Read the model definition and answer for the solid it produces. Units are mm, in the model's axes. A direction names the side the tool comes from. Round coordinates to 2 decimals unless told otherwise and drop trailing zeros. Loops run counter-clockwise (first coordinate to the right, second up) from the corner with the lowest first, then second, coordinate; pieces in that order, holes last. Notation, with made-up numbers: M 87.25,-1 L 99.25,-1 A15 cw 99.25,8 Z; hole C -29,18 d5. An arc over 180 degrees is marked long. Write each question's results on one line, items separated by ' | '.
from build123d import *

# Parameters (mm, degrees)
ESQUISSE3_W        = 75
ESQUISSE3_H        = 60
BOSS_EXTRU_4_DEPTH = 2
ESQUISSE7_R        = 3
ESQUISSE7_R_2      = 1
BOSS_EXTRU_5_DEPTH = 7


with BuildPart() as part:
    # Esquisse3 → Boss.-Extru.4 (new body)
    with BuildSketch(Plane.XY):
        Rectangle(ESQUISSE3_W, ESQUISSE3_H)
    extrude(amount=BOSS_EXTRU_4_DEPTH)

    # Esquisse7 → Boss.-Extru.5 (add)
    with BuildSketch(Plane.XY.offset(2)):
        with Locations((-17, 13.6)):
            Circle(ESQUISSE7_R)
        with Locations((17, 13.6)):
            Circle(ESQUISSE7_R)
        with Locations((7.649218941, -7.4)):
            Circle(ESQUISSE7_R_2)
    extrude(amount=BOSS_EXTRU_5_DEPTH)


solid = part.part
Item 1: The mould has two halves that part along X. Classify faces 1 (the face through (-17.391, 16.574, 5.451)), 2 (the face through (16.609, 16.574, 5.451)), 3 (the face through (17, 14, 9)), 4 (the face through (37.5, 0, 1)): pulls with the +X half, pulls with the -X half, needs draft (parallel to the pull), parting line crosses it, or undercut.
Outcome:
face 1: undercut | face 2: undercut | face 3: needs draft | face 4: pulls with the +X half
Item 2: The part is cut by section B-B (x = -17). Determine the outline of the cut face in (y, z), plus the area to 3 significant figures.
Outcome:
outline: M -30,0 L 30,0 L 30,2 L 16.6,2 L 16.6,9 L 10.6,9 L 10.6,2 L -30,2 Z | area: 162 mm2
Item 3: For faces 5 (the face through (7.52, -6.41, 5.45)), 6 (the face through (-37.5, 0, 1)), determine the directions among +Z, -Z, +X, -X, +Y, -Y from which every point of the face is accessible in a straight line to the end or side of a thin tool.
Outcome:
face 5: +Z | face 6: +Z, -Z, -X, +Y, -Y
Item 4: Straight lines are drawn through the part: line 1 (Z direction, x = 8, y = -21.5); line 2 (X direction, y = 13, z = 5.5); line 3 (Y direction, x = 19, z = 4.25). For each, find the intervals that lie inside material, in ascending order.
Outcome:
line 1: z = 0 to 2 | line 2: x = -19.94 to -14.06, 14.06 to 19.94 | line 3: y = 11.36 to 15.84
Item 5: A flat-ended cylindrical pin translates along its axis: pin 1 (3 mm diameter, centred on x = 5.5, z = 7, fed in from -Y). Find the tip coordinate at first contact, or state that the pin passes through.
Outcome:
pin 1: stops at y = -8.16
Item 6: The part is cut by section D-D (y = 13.6). Determine the outline of the cut face in (x, z).
Outcome:
outline: M -37.5,0 L 37.5,0 L 37.5,2 L 20,2 L 20,9 L 14,9 L 14,2 L -14,2 L -14,9 L -20,9 L -20,2 L -37.5,2 Z
Item 7: The part is cut by section A-A (y = -7.4). Determine the outline of the cut face in (x, z).
Outcome:
outline: M -37.5,0 L 37.5,0 L 37.5,2 L 8.65,2 L 8.65,9 L 6.65,9 L 6.65,2 L -37.5,2 Z
Item 8: The part is cut by section C-C (z = 3.5). Determine the outline of the cut face in (x, y).
Outcome:
outline: C -17,13.6 d6; C 7.65,-7.4 d2; C 17,13.6 d6
